Geometry: final body of the model. Coordinates: model frame, mm. Face numbers are marked on the shaded views. Give positions to 0.01 mm unless a question says otherwise; leave off trailing zeros. Write each loop counter-clockwise with the first axis right and the second up, starting at its lowest first coordinate (ties: lowest second). Pieces come first, ordered by that corner, then holes. Notation, with made-up numbers: M 50,24 L 87,24 A20 cw 87,59 Z; hole C -29.5,67.5 d5. An arc over 180 degrees is marked long. Use a Markdown table: item, result. Add a question column.
1) Pin query (flat end, axial travel): pin 1 (12 mm diameter, centred on x = 3.5, y = 6, fed in from +Z); pin 2 (3 mm diameter, centred on y = -6, z = 6, fed in from -X). Return the tip coordinate at first contact, or that it passes through.
2) Draft query along Y for the marked faces 1, 2 and 3. Return one class per face: +Y half, -Y half, draft (parallel to the pull), parting line (faces both ways), or undercut.
3) Section C-C on z = 6.25. Return the cut outline in (x, y).
4) Line query: line 1 (X direction, y = 11.5, z = 5.5); line 2 (Z direction, x = 11.75, y = -7); line 3 (Y direction, x = 1, z = 5.75). Output: solid intervals per line, ascending.
5) Section D-D on x = 4.5. Return the cut outline in (y, z), then the cut area to 3 significant figures.
6) Section B-B on y = 2.75. Return the cut outline in (x, z), then the cut area to 3 significant figures.
7) Section A-A on y = -9.5. Return the cut outline in (x, z), then the cut area to 3 significant figures.
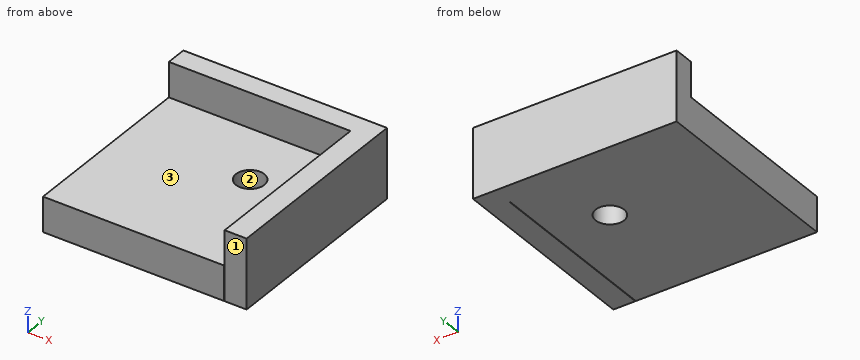
```python
from build123d import *

# Parameters (mm, degrees)
F0_W     = 26
F0_H     = 3
F1_DEPTH = 10
F0_H_2   = 26
F0_R     = 2.04741
F2_DEPTH = 5


with BuildPart() as f1:
    # F0 (on Top) → F1 (new body)
    with BuildSketch(Plane.XY):
        Polygon((12.966245, 13), (13.033755, 13), (13.033755, -13), (16.189865, -13), (16.189865, 16), (12.966245, 16), align=None)
        with Locations((-0.033755, 14.5)):
            Rectangle(F0_W, F0_H)
    extrude(amount=F1_DEPTH)

    # F0 (on Top) → F2 (join)
    with BuildSketch(Plane.XY):
        with Locations((-0.033755, 0)):
            Rectangle(F0_W, F0_H_2)
        with Locations((4.918835, 3.95259)):
            Circle(F0_R, mode=Mode.SUBTRACT)
    extrude(amount=F2_DEPTH)


solid = f1.part
```
Found:
| question | item | result |
|---|---|---|
| 1 | pin 1 | z = 5 |
| 1 | pin 2 | x = -13.03 |
| 2 | face 1 | -Y half |
| 2 | face 2 | undercut |
| 2 | face 3 | draft |
| 3 | outline | M -13.03,13 L 13.03,13 L 13.03,-13 L 16.19,-13 L 16.19,16 L -13.03,16 Z |
| 4 | line 1 | 13.03 to 16.19 |
| 4 | line 2 | 0 to 5 |
| 4 | line 3 | 13 to 16 |
| 5 | outline | M -13,0 L 1.95,0 L 1.95,5 L -13,5 Z; M 5.96,0 L 16,0 L 16,10 L 13,10 L 13,5 L 5.96,5 Z |
| 5 | area | 140 mm² |
| 6 | outline | M -13.03,0 L 3.26,0 L 3.26,5 L -13.03,5 Z; M 6.58,0 L 12.97,0 L 12.97,5 L 6.58,5 Z; M 13.03,0 L 16.19,0 L 16.19,10 L 13.03,10 Z |
| 6 | area | 145 mm² |
| 7 | outline | M -13.03,0 L 12.97,0 L 12.97,5 L -13.03,5 Z; M 13.03,0 L 16.19,0 L 16.19,10 L 13.03,10 Z |
| 7 | area | 162 mm² |
